Design review of the part built by this model. Coordinates are the model's own, in mm. A direction names the side the tool comes from. Coordinates: 2 decimals unless noted, no trailing zeros. Write each loop counter-clockwise with the first axis right and the second up, starting at its lowest first coordinate (ties: lowest second). Pieces come first, ordered by that corner, then holes. Notation, with made-up numbers: (0, 62.25) - (17, 62.25) arc R21 cw to (17, 67.25) - close; hole circle Ø11 at (49, 66.25). An arc over 180 degrees is marked (long way). Use a Markdown table: item, result.
from build123d import *

# Parameters (mm, degrees)
SKETCH1_W           = 174
SKETCH1_H           = 64
SKETCH1_W_2         = 170
SKETCH1_H_2         = 60
BOSS_EXTRUDE1_DEPTH = 25
SKETCH2_W           = 174
SKETCH2_H           = 2
BOSS_EXTRUDE2_DEPTH = 64
SKETCH9_W           = 10
SKETCH9_H           = 15
SKETCH9_R           = 2.5
BOSS_EXTRUDE3_DEPTH = 5
SKETCH10_W          = 20
SKETCH10_H          = 15
CUT_EXTRUDE2_DEPTH  = 174
CUT_EXTRUDE3_REACH  = 4
SKETCH11_R          = 2.5
SKETCH11_R_2        = 1.25


with BuildPart() as part:
    # Sketch1 → Boss-Extrude1 (new body, symmetric)
    with BuildSketch(Plane(origin=(0, 0, 0), x_dir=(1, 0, 0), z_dir=(0, 1, 0))):
        Rectangle(SKETCH1_W, SKETCH1_H)
        Rectangle(SKETCH1_W_2, SKETCH1_H_2, mode=Mode.SUBTRACT)
    extrude(amount=BOSS_EXTRUDE1_DEPTH, both=True)

    # Sketch2 → Boss-Extrude2 (add)
    with BuildSketch(Plane(origin=(0, 0, -32), x_dir=(-1, 0, 0), z_dir=(0, 0, -1))):
        with Locations((0, -24)):
            Rectangle(SKETCH2_W, SKETCH2_H)
    extrude(amount=-BOSS_EXTRUDE2_DEPTH)

    # Sketch9 → Boss-Extrude3 (add)
    with BuildSketch(Plane(origin=(0, 25, 0), x_dir=(1, 0, 0), z_dir=(0, 1, 0))):
        with Locations((-92, 0)):
            Rectangle(SKETCH9_W, SKETCH9_H)
        with Locations((-92, 0)):
            Circle(SKETCH9_R, mode=Mode.SUBTRACT)
        with Locations((92, 0)):
            Rectangle(SKETCH9_W, SKETCH9_H)
        with Locations((92, 0)):
            Circle(SKETCH9_R, mode=Mode.SUBTRACT)
    extrude(amount=-BOSS_EXTRUDE3_DEPTH)

    # Sketch10 → Cut-Extrude2 (cut)
    with BuildSketch(Plane.ZY.offset(87)):
        with Locations((0, -15.5)):
            Rectangle(SKETCH10_W, SKETCH10_H)
    extrude(amount=-CUT_EXTRUDE2_DEPTH, mode=Mode.SUBTRACT)

    # Sketch11 → Cut-Extrude3 (cut, up to next)
    with BuildSketch(Plane(origin=(0, -23, 0), x_dir=(1, 0, 0), z_dir=(0, 1, 0)), mode=Mode.PRIVATE) as cut_extrude3_sk1:
        Circle(SKETCH11_R)
    cut_extrude3_tool1 = extrude(cut_extrude3_sk1.sketch, amount=-CUT_EXTRUDE3_REACH, mode=Mode.PRIVATE) & part.part
    add(cut_extrude3_tool1.solids().sort_by_distance((0, -23, 0))[0], mode=Mode.SUBTRACT)
    # Sketch11 → Cut-Extrude3 (cut, up to next)
    with BuildSketch(Plane(origin=(0, -23, 0), x_dir=(1, 0, 0), z_dir=(0, 1, 0)), mode=Mode.PRIVATE) as cut_extrude3_sk2:
        with Locations((-41.5, 14)):
            Circle(SKETCH11_R_2)
    cut_extrude3_tool2 = extrude(cut_extrude3_sk2.sketch, amount=-CUT_EXTRUDE3_REACH, mode=Mode.PRIVATE) & part.part
    add(cut_extrude3_tool2.solids().sort_by_distance((-41.5, -23, -14))[0], mode=Mode.SUBTRACT)
    # Sketch11 → Cut-Extrude3 (cut, up to next)
    with BuildSketch(Plane(origin=(0, -23, 0), x_dir=(1, 0, 0), z_dir=(0, 1, 0)), mode=Mode.PRIVATE) as cut_extrude3_sk3:
        with Locations((-41.5, -14)):
            Circle(SKETCH11_R_2)
    cut_extrude3_tool3 = extrude(cut_extrude3_sk3.sketch, amount=-CUT_EXTRUDE3_REACH, mode=Mode.PRIVATE) & part.part
    add(cut_extrude3_tool3.solids().sort_by_distance((-41.5, -23, 14))[0], mode=Mode.SUBTRACT)


solid = part.part
(1) For L1, parallel to X at y = 23.7, z = 0; L2, parallel to Z at x = 14, y = 4; L3, parallel to X at y = 15.5, z = -1, list the stretches that pass through material, from the lowest coordinate up. Write a range as from..to.
Determined:
| item | result |
|---|---|
| L1 | -97..-94.5, -89.5..-85, 85..89.5, 94.5..97 |
| L2 | -32..-30, 30..32 |
| L3 | -87..-85, 85..87 |
(2) Take a section at A-A on z = 0. Write out the cut boundary in (x, y), and give its area (3 significant figures).
Determined:
| item | result |
|---|---|
| outline | (-97, 20) - (-94.5, 20) - (-94.5, 25) - (-97, 25) - close; (-89.5, 20) - (-87, 20) - (-87, -8) - (-85, -8) - (-85, 25) - (-89.5, 25) - close; (-87, -25) - (-2.5, -25) - (-2.5, -23) - (-87, -23) - close; (2.5, -25) - (87, -25) - (87, -23) - (2.5, -23) - close; (85, -8) - (87, -8) - (87, 20) - (89.5, 20) - (89.5, 25) - (85, 25) - close; (94.5, 20) - (97, 20) - (97, 25) - (94.5, 25) - close |
| area | 520 mm2 |
(3) Machinability: for faces 4 (the flat face through (-1, 1, -30)), 5 (the flat face through (-92, 23, 7.5)), 6 (the cylindrical face through (-94.5, 22.5, -0.1)), 7 (the flat face through (92, 23, 7.5)), which of the approach directions +Z, -Z, +X, -X, +Y, -Y give a long, thin tool a straight path to every point of the face, cutting with its end or side? Answer none if there is none.
Determined:
| item | result |
|---|---|
| face 4 | +Y |
| face 5 | +Z, -X, +Y, -Y |
| face 6 | +Y, -Y |
| face 7 | +Z, +X, +Y, -Y |
(4) Take a section at B-B on y = -15. Write out the cut boundary in (x, z).
Determined:
| item | result |
|---|---|
| outline | (-87, -32) - (87, -32) - (87, -10) - (85, -10) - (85, -30) - (-85, -30) - (-85, -10) - (-87, -10) - close; (-87, 10) - (-85, 10) - (-85, 30) - (85, 30) - (85, 10) - (87, 10) - (87, 32) - (-87, 32) - close |
(5) Take a section at C-C on x = 92. Write out the cut boundary in (y, z), and give its area (3 significant figures).
Determined:
| item | result |
|---|---|
| outline | (20, -7.5) - (25, -7.5) - (25, -2.5) - (20, -2.5) - close; (20, 2.5) - (25, 2.5) - (25, 7.5) - (20, 7.5) - close |
| area | 50.0 mm2 |
(6) For pin 1 (11 mm diameter, centred on x = -93, z = -0.5, fed in from -Y); pin 2 (24 mm diameter, centred on y = -8, z = 8.5, fed in from +X); pin 3 (5.5 mm diameter, centred on x = -94.5, y = 22, fed in from +Z), all flat-tipped, find the tip position at first contact; note any pin that passes through.
Determined:
| item | result |
|---|---|
| pin 1 | y = 20 |
| pin 2 | x = 87 |
| pin 3 | z = 7.5 |
(7) Draft analysis for pull direction Z (two halves, no side actions). For faces 1 (the flat face through (-92, 23, -7.5)), 2 (the flat face through (-85, 1, 0)), 3 (the flat face through (97, 23, 0)), state which applies: +Z half, -Z half, draft (parallel to the pull), parting line (faces both ways), or undercut.
Determined:
| item | result |
|---|---|
| face 1 | -Z half |
| face 2 | undercut |
| face 3 | draft |
(8) Take a section at D-D on y = 11. Write out the cut boundary in (x, z), and give its area (3 significant figures).
Determined:
| item | result |
|---|---|
| outline | (-87, -32) - (87, -32) - (87, 32) - (-87, 32) - close; hole (-85, -30) - (85, -30) - (85, 30) - (-85, 30) - close |
| area | 936 mm2 |
